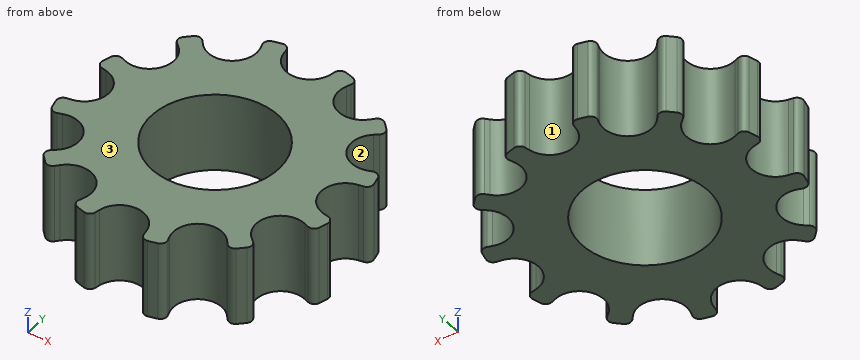
```python
from build123d import *

# Parameters (mm, degrees)
SKETCH_3_R                       = 8.977796586
EXTRUDE_2_DEPTH                  = 2.5
CUT_EXTRUDE_2_DEPTH              = 13.940311552
FILLET_1_R                       = 0.4
PATTERN_CIRCULAR_1_COUNT         = 12
FILLET_1_OF_PATTERN_CIRCULAR_1_R = 0.4
SKETCH_4_R                       = 4
CUT_EXTRUDE_3_DEPTH              = 14.348503998


with BuildPart() as part:
    # Sketch 3 → Extrude 2 (new, symmetric)
    with BuildSketch(Plane.XY):
        Circle(SKETCH_3_R)
    extrude(amount=EXTRUDE_2_DEPTH, both=True)

    # Sketch 3_3 → Cut-Extrude 2 (cut, symmetric)
    with BuildSketch(Plane.XY):
        with BuildLine():
            Line((-1.638089976, 8.827088578), (-1.509232342, 8.132720278))
            ThreePointArc((-1.509232342, 8.132720278), (0, 6.877796586), (1.509232342, 8.132720278))
            Line((1.509232342, 8.132720278), (1.638089976, 8.827088578))
            ThreePointArc((1.638089976, 8.827088578), (0, 8.977796586), (-1.638089976, 8.827088578))
        make_face()
    cut_extrude_2 = extrude(amount=CUT_EXTRUDE_2_DEPTH, both=True, mode=Mode.SUBTRACT)

    # Fillet 1
    fillet_1_edges = [part.edges().sort_by_distance(p)[0] for p in [
        (-1.638089976, 8.827088578, 0),
        (1.638089976, 8.827088578, 0),
    ]]
    fillet(fillet_1_edges, radius=FILLET_1_R)

    # Pattern Circular 1: Cut-Extrude 2 ×12 about axis
    pattern_circular_1_axis = Axis((0, 0, 0), (0, 0, 1))
    for i in range(1, PATTERN_CIRCULAR_1_COUNT):
        add(cut_extrude_2.rotate(pattern_circular_1_axis, i * 360 / PATTERN_CIRCULAR_1_COUNT), mode=Mode.SUBTRACT)

    # Fillet 1 of Pattern Circular 1
    fillet_1_of_pattern_circular_1_edges = [part.edges().sort_by_distance(p)[0] for p in [
        (-5.832171822, 6.825437962, 0),
        (-2.994916756, 8.463527938, 0),
        (-8.463527938, 2.994916756, 0),
        (-6.825437962, 5.832171822, 0),
        (-8.827088578, -1.638089976, 0),
        (-8.827088578, 1.638089976, 0),
        (-6.825437962, -5.832171822, 0),
        (-8.463527938, -2.994916756, 0),
        (-2.994916756, -8.463527938, 0),
        (-5.832171822, -6.825437962, 0),
        (1.638089976, -8.827088578, 0),
        (-1.638089976, -8.827088578, 0),
        (5.832171822, -6.825437962, 0),
        (2.994916756, -8.463527938, 0),
        (8.463527938, -2.994916756, 0),
        (6.825437962, -5.832171822, 0),
        (8.827088578, 1.638089976, 0),
        (8.827088578, -1.638089976, 0),
        (6.825437962, 5.832171822, 0),
        (8.463527938, 2.994916756, 0),
        (2.994916756, 8.463527938, 0),
        (5.832171822, 6.825437962, 0),
    ]]
    fillet(fillet_1_of_pattern_circular_1_edges, radius=FILLET_1_OF_PATTERN_CIRCULAR_1_R)

    # Sketch 4 → Cut-Extrude 3 (cut, through all)
    with BuildSketch(Plane(origin=(0, 0, -2.5), x_dir=(-1, 0, 0), z_dir=(0, 0, -1))):
        Circle(SKETCH_4_R)
    extrude(amount=-CUT_EXTRUDE_3_DEPTH, mode=Mode.SUBTRACT)


solid = part.part
```
Work out the finished part from the listing and answer in its coordinate system (mm). Face numbers are marked on the shaded views. Give positions to 0.01 mm unless a question says otherwise; leave off trailing zeros. Loops run counter-clockwise (first coordinate to the right, second up) from the corner with the lowest first, then second, coordinate; pieces in that order, holes last. Notation, with made-up numbers: M 29.25,0.5 L 74.25,0.5 A16 cw 74.25,19.5 Z; hole C 42.25,1 d2. An arc over 180 degrees is marked long. One line per item, written item: value. Start each with the question number.
1. Find section C-C (x = -4.5). Give the vertices of the cut face in (y, z).
2. Find the intervals of material crossed by probe 1 along Y at (x, z) = (0, 0.6); probe 2 along X at (y, z) = (2.5, -1.15); probe 3 along X at (y, z) = (-8, 2.25), in increasing order.
3. Each of these flat-tipped pins is pushed along its axis until it touches: P1, Ø2, axis at y = 0, z = -2, coming from the -X side; P2, Ø1.5, axis at x = 5, z = 1.5, coming from the +Y side. Where does it stop, or does it pass through?
4. Find section A-A (x = 0). Give the vertices of the cut face in (y, z).
5. Find section D-D (y = -4.75). Give the vertices of the cut face in (x, z), and give its area (3 significant figures).
6. Determine the mould class of the marked faces 1, 2 and 3 for opening direction Y: released by +Y, released by -Y, zero draft, split by the parting line, or undercut.
Reported:
1. outline: M -5.78,-2.5 L 5.78,-2.5 L 5.78,2.5 L -5.78,2.5 Z
2. probe 1: y = -6.88 to -4, 4 to 6.88
2. probe 2: x = -8.62 to -3.12, 3.12 to 8.62
2. probe 3: x = -2.83 to -1.48, 1.48 to 2.83
3. P1: stops at x = -7.25
3. P2: stops at y = 6.64
4. outline: M -6.88,-2.5 L -4,-2.5 L -4,2.5 L -6.88,2.5 Z; M 4,-2.5 L 6.88,-2.5 L 6.88,2.5 L 4,2.5 Z
5. outline: M -5.85,-2.5 L 5.85,-2.5 L 5.85,2.5 L -5.85,2.5 Z
5. area: 58.5 mm²
6. face 1: released by +Y
6. face 2: undercut
6. face 3: zero draft
